Read the model definition and answer for the solid it produces. Units are mm, in the model's axes. Face numbers are marked on the shaded views. A direction names the side the tool comes from. Give positions to 0.01 mm unless a question says otherwise; leave off trailing zeros. Order: outer loops, then holes, each group sorted by start corner. A loop starts at its lowest first (then second) coordinate and runs counter-clockwise, first axis right, second up. Notation, with made-up numbers: (33.5, 23.5) - (58.5, 23.5) arc R25 cw to (58.5, 49.5) - close; hole circle Ø1 at (88.25, -1.75). An arc over 180 degrees is marked (long way). Return JSON: item names as keys, results as strings.
```python
from build123d import *

# Parameters (mm, degrees)
F0_W     = 26.5
F0_H     = 25.5
F1_DEPTH = 98
F2_T     = -2
F4_D     = 18
F5_W     = 16
F5_H     = 18
F6_DEPTH = 2
F7_R     = 5


with BuildPart() as f1:
    # F0 (on Top) → F1 (new body)
    with BuildSketch(Plane.XY):
        Rectangle(F0_W, F0_H)
    extrude(amount=-F1_DEPTH)

    # F2
    f2_openings = [f1.faces().sort_by_distance(p)[0] for p in [
        (0, 0, 0),
    ]]
    offset(amount=F2_T, openings=f2_openings)

    # F4 (through all)
    with Locations(Plane.XY):
        with Locations((0, 0)):
            Hole(F4_D / 2)

    # F5 (on face) → F6 (cut)
    with BuildSketch(Plane.XZ.offset(12.75)):
        with Locations((0, -15.051324)):
            Rectangle(F5_W, F5_H)
    extrude(amount=-F6_DEPTH, mode=Mode.SUBTRACT)

    # F7
    f7_edges = [f1.edges().sort_by_distance(p)[0] for p in [
        (13.25, -12.75, -49),
        (13.25, 12.75, -49),
        (-13.25, -12.75, -49),
        (-13.25, 12.75, -49),
    ]]
    fillet(f7_edges, radius=F7_R)


solid = f1.part
```
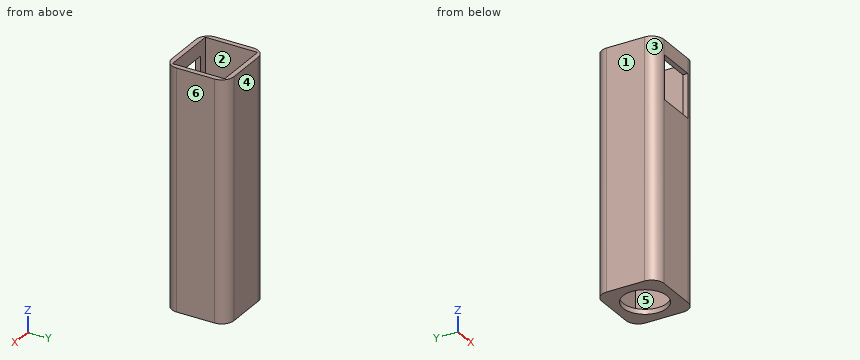
Q1. Consider L1, parallel to Y at x = 0, z = -96.65; L2, parallel to X at y = 4, z = -46.5; L3, parallel to Y at x = -3.5, z = -66. Determine where each line is inside the solid, lowest interval first.
Values:
{"L1": "y = -12.75 to -9, 9 to 12.75", "L2": "x = -13.25 to -11.25, 11.25 to 13.25", "L3": "y = -12.75 to -10.75, 10.75 to 12.75"}
Q2. For the marked faces 1 and 2, determine the directions among +Z, -Z, +X, -X, +Y, -Y from which every point of the face is accessible in a straight line to the end or side of a thin tool.
Values:
{"face 1": "+Z, -Z, -X, +Y, -Y", "face 2": "+Z"}
Q3. A cutting plane is placed at B-B (z = -46). Write down the section's boundary in (x, y).
Values:
{"outline": "(-13.25, -7.75) arc R5 ccw to (-8.25, -12.75) - (8.25, -12.75) arc R5 ccw to (13.25, -7.75) - (13.25, 7.75) arc R5 ccw to (8.25, 12.75) - (-8.25, 12.75) arc R5 ccw to (-13.25, 7.75) - close; hole (-11.25, -10.75) - (11.25, -10.75) - (11.25, 10.75) - (-11.25, 10.75) - close"}
Q4. A cutting plane is placed at A-A (x = 0). Write down the section's boundary in (y, z), and give its area (3 significant figures).
Values:
{"outline": "(-12.75, -98) - (-9, -98) - (-9, -96) - (-10.75, -96) - (-10.75, -24.05) - (-12.75, -24.05) - close; (-12.75, -6.05) - (-10.75, -6.05) - (-10.75, 0) - (-12.75, 0) - close; (9, -98) - (12.75, -98) - (12.75, 0) - (10.75, 0) - (10.75, -96) - (9, -96) - close", "area": "363 mm²"}
Q5. Determine the mould class of the marked faces 3, 4, 5 and 6 for opening direction X: released by +X, released by -X, zero draft, split by the parting line, or undercut.
Values:
{"face 3": "released by -X", "face 4": "zero draft", "face 5": "undercut", "face 6": "released by +X"}
Q6. A cutting plane is placed at C-C (y = 0). Write down the section's boundary in (x, z).
Values:
{"outline": "(-13.25, -98) - (-9, -98) - (-9, -96) - (-11.25, -96) - (-11.25, 0) - (-13.25, 0) - close; (9, -98) - (13.25, -98) - (13.25, 0) - (11.25, 0) - (11.25, -96) - (9, -96) - close"}
Q7. A cutting plane is placed at D-D (x = 4). Write down the section's boundary in (y, z), and give its area (3 significant figures).
Values:
{"outline": "(-12.75, -98) - (-8.06, -98) - (-8.06, -96) - (-10.75, -96) - (-10.75, -24.05) - (-12.75, -24.05) - close; (-12.75, -6.05) - (-10.75, -6.05) - (-10.75, 0) - (-12.75, 0) - close; (8.06, -98) - (12.75, -98) - (12.75, 0) - (10.75, 0) - (10.75, -96) - (8.06, -96) - close", "area": "367 mm²"}
Q8. Given pin 1 (3 mm diameter, centred on x = 10, z = -27, fed in from -Y); pin 2 (2 mm diameter, centred on y = -12, z = -16, fed in from -X); pin 3 (4 mm diameter, centred on x = 10.5, z = -13, fed in from +Y), each flat-ended and moving along its own axis, determine where each tip first touches the part or whether it passes through.
Values:
{"pin 1": "stops at y = -12.74", "pin 2": "stops at x = -12.05", "pin 3": "stops at y = 12.74"}
